Design review of the part built by this model. Coordinates are the model's own, in mm. A direction names the side the tool comes from. Coordinates: 2 decimals unless noted, no trailing zeros. Write each loop counter-clockwise with the first axis right and the second up, starting at its lowest first coordinate (ties: lowest second). Pieces come first, ordered by that corner, then holes. Notation, with made-up numbers: (84.5, 8) - (126.5, 8) arc R16 ccw to (126.5, 12) - close; hole circle Ø4 at (50, -27). An arc over 180 degrees is marked (long way). Answer as a JSON object with one key per item and string values.
```python
from build123d import *

# Parameters (mm, degrees)
F2_DEPTH = 20.1676
F3_W     = 40.64
F3_H     = 10.16
F4_DEPTH = 5.08


with BuildPart() as f2:
    # F1 (on Top) → F2 (new body)
    with BuildSketch(Plane.XY):
        with BuildLine():
            Line((6.7323240508, 25.4), (0, 25.4))
            Line((0, 25.4), (0, -25.4))
            Line((0, -25.4), (6.988068358, -25.4))
            ThreePointArc((6.988068358, -25.4), (18.6973375399, 0.0595921557), (6.7323240508, 25.4))
        make_face()
    extrude(amount=F2_DEPTH)

    # F3 (on face) → F4 (cut)
    with BuildSketch(Plane(origin=(0, 0, 0), x_dir=(0, -1, 0), z_dir=(-1, 0, 0))):
        with Locations((-0.0762, 10.0838)):
            Rectangle(F3_W, F3_H)
    extrude(amount=-F4_DEPTH, mode=Mode.SUBTRACT)


solid = f2.part
```
(1) For pin 1 (2 mm diameter, centred on y = -11, z = 7.5, fed in from +X); pin 2 (2 mm diameter, centred on y = -1.5, z = 13.5, fed in from +X); pin 3 (5 mm diameter, centred on y = -7.5, z = 9.5, fed in from -X), all flat-tipped, find the tip position at first contact; note any pin that passes through.
Solved:
{"pin 1": "stops at x = 17.19", "pin 2": "stops at x = 18.7", "pin 3": "stops at x = 5.08"}
(2) Take a section at C-C, the plane y = 16.5. Write out the cut boundary in (x, z), and give its area (3 significant figures).
Solved:
{"outline": "(0, 0) - (14.24, 0) - (14.24, 20.17) - (0, 20.17) - (0, 15.16) - (5.08, 15.16) - (5.08, 5) - (0, 5) - close", "area": "236 mm^2"}
(3) Take a section at B-B, the plane x = 4.5. Write out the cut boundary in (y, z).
Solved:
{"outline": "(-25.4, 0) - (25.4, 0) - (25.4, 20.17) - (-25.4, 20.17) - close; hole (-20.24, 5) - (20.4, 5) - (20.4, 15.16) - (-20.24, 15.16) - close"}
(4) Take a section at D-D, the plane x = 17.25. Write out the cut boundary in (y, z).
Solved:
{"outline": "(-9.8, 0) - (9.59, 0) - (9.59, 20.17) - (-9.8, 20.17) - close"}
(5) Tool access review of faces 1 (the face through (3, 0, 15.164)), 2 (the face through (7, 0, 0)): name each direction out of +Z, -Z, +X, -X, +Y, -Y from which nothing blocks a thin tool from reaching the whole face with its end or side.
Solved:
{"face 1": "-X", "face 2": "-Z, +X, -X, +Y, -Y"}
(6) The part is to be moulded in two halves that separate along Y. For faces 3 (the face through (3, 25.4, 10)), 4 (the face through (3, -25.4, 10)), 5 (the face through (3, 0, 5.004)), 6 (the face through (18.697, -0.345, 9.943)), say which applies: pulls with the +Y half, pulls with the -Y half, needs draft (parallel to the pull), parting line crosses it, or undercut.
Solved:
{"face 3": "pulls with the +Y half", "face 4": "pulls with the -Y half", "face 5": "undercut", "face 6": "parting line crosses it"}
(7) Take a section at A-A, the plane z = 13.5. Write out the cut boundary in (x, y).
Solved:
{"outline": "(0, -25.4) - (6.99, -25.4) arc R33.17 ccw to (6.73, 25.4) - (0, 25.4) - (0, 20.4) - (5.08, 20.4) - (5.08, -20.24) - (0, -20.24) - close"}
(8) To check wall thickness, follow line 1 (Z direction, x = 1.75, y = -16); line 2 (Y direction, x = 3.75, z = 7.5); line 3 (X direction, y = -0.5, z = 8.5). State the ranges of each line that lie inside material, in increasing order. Write a range as from..to.
Solved:
{"line 1": "z = 0..5, 15.16..20.17", "line 2": "y = -25.4..-20.24, 20.4..25.4", "line 3": "x = 5.08..18.7"}
